from build123d import *

# Parameters (mm, degrees)
BOSS_EXTRUDE1_DEPTH = 3


with BuildPart() as part:
    # Sketch1 → Boss-Extrude1 (new body)
    with BuildSketch(Plane(origin=(0, 0, 0), x_dir=(0, 0, -1), z_dir=(1, 0, 0))):
        with BuildLine():
            Line((16.10495, 157.49285), (16.10495, 160.49285))
            Line((16.10495, 160.49285), (-15.93645, 160.49285))
            Line((-15.93645, 160.49285), (-15.93645, 157.49285))
            Line((-15.93645, 157.49285), (-265.87855, 157.49285))
            Line((-265.87855, 157.49285), (-282.48125, 128.79465))
            Line((-282.48125, 128.79465), (-295.04705, 136.06965))
            Line((-295.04705, 136.06965), (-308.92005, 112.09525))
            Line((-308.92005, 112.09525), (-296.35425, 104.81525))
            Line((-296.35425, 104.81525), (-314.21085, 73.95765))
            Line((-314.21085, 73.95765), (-537.85245, -5.03885))
            Line((-537.85245, -5.03885), (-500.83535, -63.92765))
            Line((-500.83535, -63.92765), (-529.90705, -82.29115))
            add(Edge.make_bspline(
                [(-529.90705, -82.29115), (-538.09755, -87.38345), (-540.60535, -98.15845), (-535.50965, -106.34895)],
                knots=[0, 0, 0, 0, 1, 1, 1, 1], degree=3))
            add(Edge.make_bspline(
                [(-535.50965, -106.34895), (-530.41395, -114.53935), (-519.64405, -117.04885), (-511.45355, -111.94645)],
                knots=[0, 0, 0, 0, 1, 1, 1, 1], degree=3))
            Line((-511.45355, -111.94645), (-482.27845, -93.44795))
            Line((-482.27845, -93.44795), (-445.30805, -152.26515))
            Line((-445.30805, -152.26515), (-182.28825, -152.26515))
            Line((-182.28825, -152.26515), (-182.28825, -155.26515))
            Line((-182.28825, -155.26515), (-85.48695, -155.26515))
            Line((-85.48695, -155.26515), (-85.48695, -152.26515))
            Line((-85.48695, -152.26515), (311.39965, -152.26515))
            Line((311.39965, -152.26515), (311.39965, -155.26515))
            Line((311.39965, -155.26515), (408.19765, -155.26515))
            Line((408.19765, -155.26515), (408.19765, -152.26515))
            Line((408.19765, -152.26515), (539.35145, -152.26515))
            Line((539.35145, -152.26515), (539.35145, -118.55455))
            Line((539.35145, -118.55455), (492.29645, -118.55455))
            Line((492.29645, -118.55455), (492.29645, -65.31325))
            Line((492.29645, -65.31325), (506.80985, -65.31325))
            Line((506.80985, -65.31325), (506.80985, 79.88545))
            Line((506.80985, 79.88545), (492.28815, 79.88545))
            Line((492.28815, 79.88545), (492.28815, 133.13165))
            Line((492.28815, 133.13165), (535.57645, 133.13165))
            Line((535.57645, 133.13165), (535.76985, 157.49285))
            Line((535.76985, 157.49285), (306.50565, 157.49285))
            Line((306.50565, 157.49285), (306.50565, 160.49285))
            Line((306.50565, 160.49285), (209.70605, 160.49285))
            Line((209.70605, 160.49285), (209.70605, 157.49285))
            Line((209.70605, 157.49285), (16.10495, 157.49285))
        make_face()
        Polygon((-239.31955, 33.14975), (-103.79955, 33.14975), (-103.79955, 43.14975), (-224.79955, 43.14975), (-224.79955, 38.14975), (-239.31955, 38.14975), align=None, mode=Mode.SUBTRACT)
        Polygon((-55.93395, 66.85645), (-55.93395, -68.66355), (-45.93395, -68.66355), (-45.93395, 52.33645), (-50.93395, 52.33645), (-50.93395, 66.85645), align=None, mode=Mode.SUBTRACT)
        Polygon((-372.99945, 28.80995), (-372.99945, -106.71005), (-362.99945, -106.71005), (-362.99945, 14.28995), (-367.99945, 14.28995), (-367.99945, 28.80995), align=None, mode=Mode.SUBTRACT)
        Polygon((392.83665, 64.84155), (392.83665, -70.67845), (402.83665, -70.67845), (402.83665, 50.32155), (397.83665, 50.32155), (397.83665, 64.84155), align=None, mode=Mode.SUBTRACT)
        with BuildLine():
            add(Edge.make_bspline(
                [(-521.52825, -107.45275), (-527.12745, -107.45275), (-531.66795, -102.92065), (-531.66795, -97.31475)],
                knots=[0, 0, 0, 0, 0.333333333, 0.333333333, 0.333333333, 0.333333333], degree=3))
            add(Edge.make_bspline(
                [(-531.66795, -97.31475), (-531.66795, -91.71715), (-527.12915, -87.17505), (-521.52825, -87.17505)],
                knots=[0.333333333, 0.333333333, 0.333333333, 0.333333333, 1, 1, 1, 1], degree=3))
            add(Edge.make_bspline(
                [(-521.52825, -87.17505), (-515.92735, -87.17505), (-511.39025, -91.71385), (-511.39025, -97.31475)],
                knots=[0, 0, 0, 0, 0.333333333, 0.333333333, 0.333333333, 0.333333333], degree=3))
            add(Edge.make_bspline(
                [(-511.39025, -97.31475), (-511.39025, -102.92065), (-515.92895, -107.45275), (-521.52825, -107.45275)],
                knots=[0.333333333, 0.333333333, 0.333333333, 0.333333333, 1, 1, 1, 1], degree=3))
        make_face(mode=Mode.SUBTRACT)
    extrude(amount=BOSS_EXTRUDE1_DEPTH)


solid = part.part
Geometry: final body of the model. Coordinates: model frame, mm. A direction names the side the tool comes from. Round coordinates to 2 decimals unless told otherwise and drop trailing zeros. Loops run counter-clockwise (first coordinate to the right, second up) from the corner with the lowest first, then second, coordinate; pieces in that order, holes last.
Q1. Section D-D on y = -133. Return loops of the section in (x, z), plus the area to 3 significant figures.
Q2. Pin query (flat end, axial travel): P1, Ø1.5, axis at x = 2, z = -79, coming from the +Y side; P2, Ø0.9, axis at x = 1, y = -85.5, coming from the -Z side; P3, Ø0.9, axis at x = 1, z = -498, coming from the -Y side. Return the tip coordinate at first contact, or that it passes through.
Q3. Section C-C on x = 0.75. State how many separate pieces and enclosed holes the cut face has, plus the area to 3 significant figures.
Q4. Access query for faces 5 (the flat face through (1.479, -102.827, 497.07)), 6 (the flat face through (3, 5, -112)), 7 (the flat face through (1.479, -34.071, 519.603)). Directions: +Z, -Z, +X, -X, +Y, -Y. A direction counts if a zero-diameter tool reaches every point of the face in a straight line with its end or side. Return the directions, or none.
Q5. Section B-B on z = -119.5. Return loops of the section in (x, y), plus the area to 3 significant figures.
Q6. Material intervals for L1, parallel to Z at x = 1.65, y = -92.5; L2, parallel to Y at x = 2.5, z = 108.5; L3, parallel to Z at x = 0.3, y = -63, sorted ascending.
Q7. Section A-A on y = -19.5. Return loops of the section in (x, z).
Q8. Pull-direction query (Y, two-part tool) for faces 1 (the flat face through (0, 5, -112)), 2 (the flat face through (1.5, 35, 424.5)), 3 (the flat face through (1.48, 89.6, 305.16)), 4 (the flat face through (1.5, -73, 515.2)); classes: released by +Y, released by -Y, zero draft, split by the parting line, or undercut.
Evaluation:
1. outline: (0, -539.35) - (3, -539.35) - (3, 457.42) - (0, 457.42) - close
1. area: 2,990 mm2
2. P1: stops at y = 157.49
2. P2: stops at z = -492.3
2. P3: stops at y = -152.27
3. separate pieces: 1
3. enclosed holes: 5
3. area: 285,000 mm2
4. face 5: +X, -X, -Y
4. face 6: +Z, -Z, +X, +Y, -Y
4. face 7: +Z, +X, -X
5. outline: (0, -152.27) - (3, -152.27) - (3, 157.49) - (0, 157.49) - close
5. area: 929 mm2
6. L1: z = -492.3 to 363, 373 to 512.6, 530.45 to 537.52
6. L2: y = -155.27 to 33.15, 43.15 to 157.49
6. L3: z = -506.81 to -402.84, -392.84 to 45.93, 55.93 to 363, 373 to 501.42
7. outline: (0, -506.81) - (3, -506.81) - (3, -402.84) - (0, -402.84) - close; (0, -392.84) - (3, -392.84) - (3, 45.93) - (0, 45.93) - close; (0, 55.93) - (3, 55.93) - (3, 363) - (0, 363) - close; (0, 373) - (3, 373) - (3, 528.76) - (0, 528.76) - close
8. face 1: zero draft
8. face 2: released by +Y
8. face 3: undercut
8. face 4: undercut
